from build123d import *

# Parameters (mm, degrees)
F0_W     = 3.175
F0_H     = 12.7
F0_W_2   = 12.7
F0_H_2   = 3.175
F1_DEPTH = 3.175


with BuildPart() as f1:
    # F0 (on Front) → F1 (new body)
    with BuildSketch(Plane.XZ):
        Polygon((-20.32, 30.1625), (-31.75, 30.1625), (-31.75, 3.175), (-31.75, -9.525), (-31.75, -30.1625), (-6.35, -30.1625), (6.35, -30.1625), (31.75, -30.1625), (31.75, -9.525), (31.75, 3.175), (31.75, 30.1625), (20.32, 30.1625), (18.7325, 20.6375), (17.145, 30.1625), (15.5575, 20.6375), (13.97, 30.1625), (-2.54, 30.1625), (-5.715, 20.6375), (-8.89, 30.1625), (-13.97, 30.1625), (-13.97, 23.8125), (-20.32, 23.8125), align=None)
        with Locations((33.3375, -3.175)):
            Rectangle(F0_W, F0_H)
        with Locations((0, -31.75)):
            Rectangle(F0_W_2, F0_H_2)
        with Locations((-33.3375, -3.175)):
            Rectangle(F0_W, F0_H)
    extrude(amount=F1_DEPTH)


solid = f1.part
Geometry: final body of the model. Coordinates: model frame, mm. A direction names the side the tool comes from. Give positions to 0.01 mm unless a question says otherwise; leave off trailing zeros. Write each loop counter-clockwise with the first axis right and the second up, starting at its lowest first coordinate (ties: lowest second). Pieces come first, ordered by that corner, then holes.
(1) Cut plane C-C, the plane x = -25.5. Return loops of the section in (y, z) (1 decimal), then the cut area to 3 significant figures.
(2) Cut plane B-B, the plane z = 15.5. Return loops of the section in (x, y) (3 decimals).
(3) Access query for faces 4 (the flat face through (33, -2, 3.175)), 5 (the flat face through (19, -2, -30.162)), 6 (the flat face through (-4.105, -1.565, 25.467)). Directions: +Z, -Z, +X, -X, +Y, -Y. A direction counts if a zero-diameter tool reaches every point of the face in a straight line with its end or side. Return the directions, or none.
(4) Mould query, pull axis X, two halves, no side actions, for faces 1 (the flat face through (-19, -2, -30.162)), 2 (the flat face through (31.75, -2, 16)), 3 (the flat face through (-13.97, -2, 27)). Classes: released by +X, released by -X, zero draft, split by the parting line, or undercut.
(5) First-contact query: P1, Ø1, axis at x = -12.5, y = -1.5, coming from the -Z side; P2, Ø1, axis at y = -1, z = 26.5, coming from the -X side; P3, Ø1, axis at x = -33.5, y = -2, coming from the -Z side (3 decimals). Flat tips, straight axial feed; report the tip coordinate or a pass-through.
(6) Ray query, line 1 (X direction, y = -1.8, z = 27.5); line 2 (X direction, y = -2.7, z = 8); line 3 (Z direction, x = 30.5, y = -3). Return the intervals inside material, ascending.
Values follow:
1. outline: (-3.2, -30.2) - (0, -30.2) - (0, 30.2) - (-3.2, 30.2) - close
1. area: 192 mm2
2. outline: (-31.75, -3.175) - (31.75, -3.175) - (31.75, 0) - (-31.75, 0) - close
3. face 4: +Z, +X, +Y, -Y
3. face 5: -Z, +X, +Y, -Y
3. face 6: +Z, +Y, -Y
4. face 1: zero draft
4. face 2: released by +X
4. face 3: undercut
5. P1: stops at z = -30.16
5. P2: stops at x = -31.75
5. P3: stops at z = -9.525
6. line 1: x = -31.75 to -20.32, -13.97 to -8, -3.43 to 14.41, 16.7 to 17.59, 19.88 to 31.75
6. line 2: x = -31.75 to 31.75
6. line 3: z = -30.16 to 30.16
